The listing builds one solid part. Answer for the finished solid, in the listing's coordinates (mm). A direction names the side the tool comes from. Give positions to 0.01 mm unless a question says otherwise; leave off trailing zeros. Loops run counter-clockwise (first coordinate to the right, second up) from the corner with the lowest first, then second, coordinate; pieces in that order, holes last. Notation, with made-up numbers: M 84.25,65 L 97.25,65 A21 cw 97.25,81 Z; hole C 54.25,-7.75 d11. An arc over 180 degrees is marked long. Use one line per item in the form item = value. Start each with the question number.
1. The part is cut by section C-C (x = 3). Write down the section's boundary in (y, z), and give its area (3 significant figures).
2. For faces 4 (the face through (7.64, -1.69, -1.84)), 5 (the face through (14.5, -4, 4)), 6 (the face through (2.62, 4.62, -1.19)), 7 (the face through (2.62, 1.19, 4.62)), determine the directions among +Z, -Z, +X, -X, +Y, -Y from which every point of the face is accessible in a straight line to the end or side of a thin tool.
3. Each of these flat-tipped pins is pushed along its axis until it touches: pin 1 Ø1 at (x, y) = (13, -2) entering from +Z; pin 2 Ø8 at (x, z) = (13.5, 3.5) entering from +Y; pin 3 Ø2 at (x, y) = (3, 0) entering from +Z; pin 4 Ø6 at (x, z) = (12, 2) entering from +Y. Where does it stop, or does it pass through?
4. The mould has two halves that part along X. Classify faces 1 (the face through (15.29, 6.21, 3.23)), 2 (the face through (7, -4, -4)), 3 (the face through (15.5, 3, 0)): released by +X, released by -X, zero draft, split by the parting line, or undercut.
5. The part is cut by section A-A (z = 0). Write down the section's boundary in (x, y), and give its area (3 significant figures).
6. Straight lines are drawn through the part: line 1 (Y direction, x = 5.5, z = 0); line 2 (X direction, y = 4.85, z = 0); line 3 (Y direction, x = 11.5, z = 0). For each, find the intervals that lie inside material, in ascending order. Write a range as from..to.
7. The part is cut by section D-D (y = 5.5). Give the number of separate pieces and of enclosed holes in the cut face, and give its area (3 significant figures).
from build123d import *

# Parameters (mm, degrees)
ESQUISSE2_W = 1.25
ESQUISSE2_H = 7
ESQUISSE5_W = 1.25
ESQUISSE5_H = 7


with BuildPart() as part:
    # Esquisse1 → Révolution1 (revolve)
    with BuildSketch(Plane.XY, mode=Mode.PRIVATE) as r_volution1_sk:
        Polygon((0, 2.5), (0, 7), (6.422649731, 7), (7, 6), (7, 5), (14.5, 5), (14.5, 6), (15.077350269, 7), (15.5, 7), (15.5, 2.5), align=None)
    revolve(r_volution1_sk.sketch.rotate(Axis((0, 0, 0), (1, 0, 0)), 90), axis=Axis((0, 0, 0), (1, 0, 0)))

    # Esquisse2 → Trou taraudé M31 (revolve, cut)
    with BuildSketch(Plane.YZ.offset(3)):
        with Locations((0.625, 3.5)):
            Rectangle(ESQUISSE2_W, ESQUISSE2_H)
    revolve(axis=Axis((3, 0, -6.35), (0, 0, 1)), mode=Mode.SUBTRACT)

    # Esquisse5 → Trou taraudé M32 (revolve, cut)
    with BuildSketch(Plane(origin=(3, 0, 0), x_dir=(0, 0, -1), z_dir=(1, 0, 0))):
        with Locations((0.625, 3.5)):
            Rectangle(ESQUISSE5_W, ESQUISSE5_H)
    revolve(axis=Axis((3, -6.35, 0), (0, 1, 0)), mode=Mode.SUBTRACT)


solid = part.part
Derived:
q1.outline = M -1.25,2.17 L -1.25,6.89 A7 ccw long 6.89,-1.25 L 2.17,-1.25 A2.5 cw long Z; M 1.25,2.17 A2.5 cw 2.17,1.25 L 6.89,1.25 A7 ccw 1.25,6.89 Z
q1.area = 111 mm2
q2.face_4 = +X, -X
q2.face_5 = none
q2.face_6 = +Y
q2.face_7 = +Z
q3.pin_1 = 4.77
q3.pin_2 = 7
q3.pin_3 = -2.29
q3.pin_4 = 6.63
q4.face_1 = zero draft
q4.face_2 = undercut
q4.face_3 = released by +X
q5.outline = M 0,-7 L 6.42,-7 L 7,-6 L 7,-5 L 14.5,-5 L 14.5,-6 L 15.08,-7 L 15.5,-7 L 15.5,-2.5 L 0,-2.5 Z; M 0,2.5 L 1.75,2.5 L 1.75,7 L 0,7 Z; M 4.25,2.5 L 15.5,2.5 L 15.5,7 L 15.08,7 L 14.5,6 L 14.5,5 L 7,5 L 7,6 L 6.42,7 L 4.25,7 Z
q5.area = 97.1 mm2
q6.line_1 = -7..-2.5, 2.5..7
q6.line_2 = 0..1.75, 4.25..15.5
q6.line_3 = -5..-2.5, 2.5..5
q7.separate_pieces = 2
q7.enclosed_holes = 1
q7.area = 62.3 mm2
